from build123d import *

# Parameters (mm, degrees)
SKETCH1_R           = 3.175
SKETCH1_R_2         = 1.5875
BOSS_EXTRUDE1_DEPTH = 2.016125
SKETCH2_R           = 3.7592
SKETCH2_R_2         = 1.5875
BOSS_EXTRUDE2_DEPTH = 0.7874
SKETCH3_R           = 2.8702
SKETCH3_R_2         = 1.9812
CUT_EXTRUDE1_DEPTH  = 0.381


with BuildPart() as part:
    # Sketch1 → Boss-Extrude1 (new body)
    with BuildSketch(Plane.XY):
        Circle(SKETCH1_R)
        Circle(SKETCH1_R_2, mode=Mode.SUBTRACT)
    extrude(amount=BOSS_EXTRUDE1_DEPTH)

    # Sketch2 → Boss-Extrude2 (add)
    with BuildSketch(Plane.XY.offset(2.016125)):
        Circle(SKETCH2_R)
        Circle(SKETCH2_R_2, mode=Mode.SUBTRACT)
    extrude(amount=BOSS_EXTRUDE2_DEPTH)

    # Sketch3 → Cut-Extrude1 (cut)
    with BuildSketch(Plane.XY.offset(2.803525)):
        Circle(SKETCH3_R)
        Circle(SKETCH3_R_2, mode=Mode.SUBTRACT)
    extrude(amount=-CUT_EXTRUDE1_DEPTH, mode=Mode.SUBTRACT)


solid = part.part
Read the model definition and answer for the solid it produces. Units are mm, in the model's axes. A direction names the side the tool comes from. Coordinates: 2 decimals unless noted, no trailing zeros. Order: outer loops, then holes, each group sorted by start corner. A loop starts at its lowest first (then second) coordinate and runs counter-clockwise, first axis right, second up. Notation, with made-up numbers: M 54.5,30 L 102.5,30 A23 ccw 102.5,55 Z; hole C 55.25,71 d8. An arc over 180 degrees is marked long. Put each result on its own line as item: value. Start each with the question number.
Item 1: Consider probe 1 along Y at (x, z) = (0, 2.65); probe 2 along Y at (x, z) = (0, 0.9) (1 decimal); probe 3 along Y at (x, z) = (0.5, 2.6). Determine where each line is inside the solid, lowest interval first. Write a range as [from, to].
Item 2: Section D-D, the plane x = -2.75 is taken. Determine the outline of the cut face in (y, z).
Item 3: The mould has two halves that part along X. Classify faces 4 (the face through (1.4, -1.4, 0)), 5 (the face through (-0.34, -1.55, 1.38)), 6 (the face through (-0.69, -3.1, 0.99)): +X half, -X half, draft (parallel to the pull), parting line (faces both ways), or undercut.
Item 4: For faces 1 (the face through (-0.258, 1.964, 2.616)), 2 (the face through (-3, -2, 2.016)), 3 (the face through (-0.81, -3.67, 2.4)), determine the directions among +Z, -Z, +X, -X, +Y, -Y from which every point of the face is accessible in a straight line to the end or side of a thin tool.
Computed:
1. probe 1: y = [-3.76, -2.87], [-1.98, -1.59], [1.59, 1.98], [2.87, 3.76]
1. probe 2: y = [-3.2, -1.6], [1.6, 3.2]
1. probe 3: y = [-3.73, -2.83], [-1.92, -1.51], [1.51, 1.92], [2.83, 3.73]
2. outline: M -2.56,2.02 L -1.59,2.02 L -1.59,0 L 1.59,0 L 1.59,2.02 L 2.56,2.02 L 2.56,2.8 L 0.82,2.8 L 0.82,2.42 L -0.82,2.42 L -0.82,2.8 L -2.56,2.8 Z
3. face 4: draft
3. face 5: undercut
3. face 6: parting line
4. face 1: +Z
4. face 2: -Z
4. face 3: +Z, -Z
